Here's how the part is built. I have some questions about the finished solid (model axes, mm). A direction names the side the tool comes from. Coordinates: 2 decimals unless noted, no trailing zeros. Write each loop counter-clockwise with the first axis right and the second up, starting at its lowest first coordinate (ties: lowest second). Pieces come first, ordered by that corner, then holes. Notation, with made-up numbers: (2.25, 73) - (11.25, 73) arc R27 ccw to (11.25, 96) - close; hole circle Ø1 at (35, 75). An arc over 180 degrees is marked (long way). Answer in a Markdown table with one row per item. Add a question column.
Item 1: Imagine slicing it at A-A (y = 3). Please give me the cut outline in (x, z).
Item 2: Imagine slicing it at C-C (x = -2.5). Please give me the cut outline in (y, z) (3 decimals).
Item 3: I'm going to push flat-ended pins straight in: pin 1 (2 mm diameter, centred on x = 3, y = 8.5, fed in from +Z); pin 2 (3.5 mm diameter, centred on y = 9.5, z = -13.5, fed in from +X); pin 3 (0.6 mm diameter, centred on x = 4.5, z = 19, fed in from -Y). Where does each tip first touch, or does it pass through?
Item 4: We'd pull the mould along Z, two halves only. Please class faces 1 (the face through (-5, 10, -11)), 2 (the face through (-4.01, 8.46, -12.01)), 3 (the face through (6, 10, 9)): +Z half, -Z half, draft (parallel to the pull), parting line (faces both ways), or undercut.
Item 5: If I drill on probe 1 along X at (y, z) = (12, 16); probe 2 along X at (y, z) = (11, -11.5); probe 3 along Z at (x, y) = (-2.2, 9.75) (3 decimals), over which ranges is the centre line in solid material (lowest first)? Write a range as from..to.
Item 6: Imagine slicing it at B-B (x = 0). Please give me the cut outline in (y, z).
Item 7: Imagine slicing it at D-D (z = -13). Please give me the cut outline in (x, y) (3 decimals).
Item 8: Which directions (+Z, -Z, +X, -X, +Y, -Y) give clear straight access to the entire face, cutting with the end or side of a thin tool? Please do faces 4 (the face through (-5, 10, 9)), 5 (the face through (1, 10, 9)), 6 (the face through (-6, 10, -9)).
Autodesk Inventor part; units mm, degrees
ref_plane "YZ Plane" through (0, 0, 0) normal (1, 0, 0) x (0, 1, 0)
ref_plane "XZ Plane" through (0, 0, 0) normal (0, 1, 0) x (-1, 0, 0)
ref_plane "XY Plane" through (0, 0, 0) normal (0, 0, 1) x (1, 0, 0)
sketch "Sketch7" plane through (0, 0, 0) normal (1, 0, 0) x (0, 1, 0)
  line L0 (-2.6, 0) -> (15.6, 0)
  line L1 (0, -24.701) -> (0, 24.701)
  line L2 (0, 2.5) -> (0, -2.5)
  line L3 (13, 15.5) -> (13, 0)
  line L4 (0, 2.5) -> (6.5, 9)
  line L5 (0, 2.5) -> (9.1924, 2.5) construction
  arc A0 (13, 15.5) -> (6.5, 9) centre (11.1419, 10.8581) ccw
  circle A1 centre (9.75, 13) radius 1.625
  line L6 (13, -15.5) -> (13, 0)
  line L7 (0, -2.5) -> (6.5, -9)
  arc A2 (6.5, -9) -> (13, -15.5) centre (11.1419, -10.8581) ccw
  circle A3 centre (9.75, -13) radius 1.625
  point P0 (0, 0)
  dimension "d64" = 5
  dimension "d65" = 2.5
  dimension "d66" = 45
  dimension "d67" = 6.5
  dimension "d68" = 13
  dimension "d69" = 15.5
  dimension "d70" = 5
  dimension "d71" = 3.25
  dimension "d74" = 3.25
  dimension "d103" = 2.5
extrude "Extrusion5" add sketch "Sketch7" along normal mid plane 13
sketch "Sketch8" plane through (-6.5, 13, 15.5) normal (0, 1, 0) x (1, 0, 0)
  line L0 (0, 6.5) -> (13, 6.5)
  line L1 (11.5, 6.5) -> (13, 6.5)
  line L2 (13, 6.5) -> (13, -0.5)
  line L3 (13, -0.5) -> (11.5, -0.5)
  line L4 (11.5, -0.5) -> (11.5, 6.5)
  line L5 (13, 31) -> (13, 0)
  line L6 (5.5, 6.5) -> (9.5, 6.5)
  line L7 (9.5, 6.5) -> (9.5, -0.5)
  line L8 (9.5, -0.5) -> (5.5, -0.5)
  line L9 (5.5, -0.5) -> (5.5, 6.5)
  line L10 (0, 6.5) -> (3.5, 6.5)
  line L11 (3.5, 6.5) -> (3.5, -0.5)
  line L12 (3.5, -0.5) -> (0, -0.5)
  line L13 (0, -0.5) -> (0, 6.5)
  line L14 (0, 0) -> (0, 31)
  point P0 (6.5, 15.5)
  dimension "d77" = 1.5
  dimension "d78" = 7
  dimension "d79" = 4
  dimension "d80" = 7
  dimension "d81" = 2
  dimension "d83" = 7
  dimension "d101" = 2
extrude "Extrusion6" cut sketch "Sketch8" against normal blind 10
sketch "Sketch9" plane through (-6.5, 13, -15.5) normal (0, 1, 0) x (1, 0, 0)
  line L0 (0, -6.5) -> (13, -6.5)
  line L1 (1.5, -6.5) -> (0, -6.5)
  line L2 (0, -6.5) -> (0, 0.5)
  line L3 (0, 0.5) -> (1.5, 0.5)
  line L4 (1.5, 0.5) -> (1.5, -6.5)
  line L5 (0, -24.5) -> (0, 0)
  line L6 (7.5, -6.5) -> (3.5, -6.5)
  line L7 (3.5, -6.5) -> (3.5, 0.5)
  line L8 (3.5, 0.5) -> (7.5, 0.5)
  line L9 (7.5, 0.5) -> (7.5, -6.5)
  line L10 (13, -6.5) -> (9.5, -6.5)
  line L11 (9.5, -6.5) -> (9.5, 0.5)
  line L12 (9.5, 0.5) -> (13, 0.5)
  line L13 (13, 0.5) -> (13, -6.5)
  line L14 (13, 0) -> (13, -24.5)
  point P0 (6.5, -15.5)
  dimension "d86" = 1.5
  dimension "d87" = 7
  dimension "d88" = 4
  dimension "d89" = 7
  dimension "d90" = 2
  dimension "d92" = 7
  dimension "d102" = 2
extrude "Extrusion7" cut sketch "Sketch9" against normal blind 10
sketch "Sketch10" plane through (1, 13, -9) normal (0, 0, -1) x (-1, 0, 0)
  line L0 (1, -15.6) -> (1, 2.6)
  line L1 (7.5, -13) -> (-5.5, -13)
  circle A0 centre (1, -3) radius 0.75
  line L2 (0, 0) -> (4, 0)
  circle A1 centre (1, -10) radius 0.75
  point P0 (1, -13)
  dimension "d95" = 1.5
  dimension "d96" = 3
  dimension "d97" = 1.5
  dimension "d98" = 3
extrude "Extrusion8" cut sketch "Sketch10" against normal blind 20
sketch "Sketch13" plane through (5, 13, 15.5) normal (1, 0, 0) x (0, 0, -1)
  line L0 (-5, 0) -> (0, 0)
  line L1 (0, 0) -> (0, -2)
  line L2 (0, -2) -> (-5, -2)
  line L3 (-5, -2) -> (-5, 0)
  line L4 (0, 0) -> (6.5, 0)
  point P0 (15.5, -13)
  dimension "d112" = 5
  dimension "d113" = 2
extrude "Extrusion11" add sketch "Sketch13" against normal blind 2
sketch "Sketch14" plane through (-3, 13, 9) normal (-1, 0, 0) x (0, 0, 1)
  line L0 (6.5, 0) -> (0, 0)
  line L1 (6.5, 0) -> (11.5, 0)
  line L2 (11.5, 0) -> (11.5, -2)
  line L3 (11.5, -2) -> (6.5, -2)
  line L4 (6.5, -2) -> (6.5, 0)
  point P0 (-9, -13)
  dimension "d116" = 5
  dimension "d117" = 2
extrude "Extrusion12" add sketch "Sketch14" against normal blind 2
properties part number "finger_joins"
Here are the results:
| question | item | result |
|---|---|---|
| 1 | outline | (-6.5, -5.5) - (-0.75, -5.5) - (-0.75, 5.5) - (-6.5, 5.5) - close; (0.75, -5.5) - (6.5, -5.5) - (6.5, 5.5) - (0.75, 5.5) - close |
| 2 | outline | (0, -2.5) - (6.5, -9) - (13, -9) - (13, 20.5) - (11, 20.5) - (11, 15.856) arc R5 ccw to (6.5, 9) - (0, 2.5) - close; hole circle Ø3.25 at (9.75, 13) |
| 3 | pin 1 | stops at z = 15.58 |
| 3 | pin 2 | stops at x = 3 |
| 3 | pin 3 | stops at y = 11 |
| 4 | face 1 | draft |
| 4 | face 2 | undercut |
| 4 | face 3 | +Z half |
| 5 | probe 1 | x = -3..-1, 3..5 |
| 5 | probe 2 | x = -5..-3, 1..3 |
| 5 | probe 3 | z = -9..11.375, 14.625..15.66 |
| 6 | outline | (0, -2.5) - (2.25, -4.75) - (2.25, 4.75) - (0, 2.5) - close; (3.75, -6.25) - (6.5, -9) - (9.25, -9) - (9.25, 9) - (6.5, 9) - (3.75, 6.25) - close; (10.75, -9) - (13, -9) - (13, 9) - (10.75, 9) - close |
| 7 | outline | (-5, 6.624) - (-3, 6.624) - (-3, 8.125) - (-5, 8.125) - close; (-5, 11.375) - (-3, 11.375) - (-3, 13) - (-5, 13) - close; (1, 6.624) - (3, 6.624) - (3, 8.125) - (1, 8.125) - close; (1, 11.375) - (3, 11.375) - (3, 13) - (1, 13) - close |
| 8 | face 4 | +Z, -X, +Y, -Y |
| 8 | face 5 | +Z, +Y, -Y |
| 8 | face 6 | -Z, -X, +Y, -Y |
